Geometry: final body of the model. Coordinates: model frame, mm. Give positions to 0.01 mm unless a question says otherwise; leave off trailing zeros. Loops run counter-clockwise (first coordinate to the right, second up) from the corner with the lowest first, then second, coordinate; pieces in that order, holes last. Notation, with made-up numbers: (34, 78) -> (68, 78) arc R11 cw to (68, 83) -> close; hole circle Ø2 at (33, 46.25). An arc over 180 degrees is marked (long way). Answer in a Markdown table with one row per item. Add a question column.
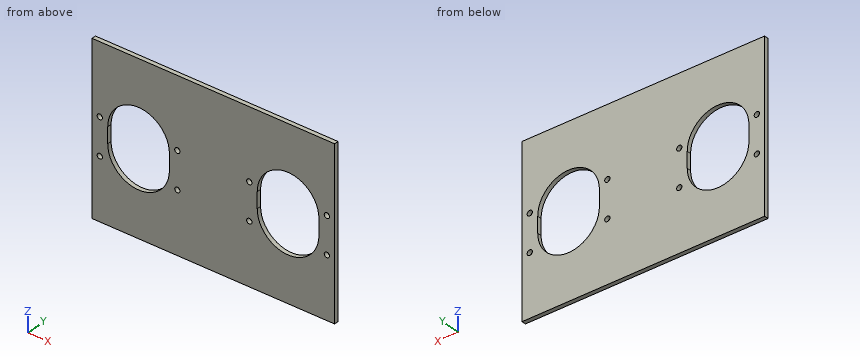
from build123d import *

# Parameters (mm, degrees)
F0_W     = 688
F0_H     = 90
F0_H_2   = 300
F0_R     = 7.5
F1_DEPTH = 12


with BuildPart() as f1:
    # F0 (on Front) → F1 (new body)
    with BuildSketch(Plane.XZ):
        with Locations((344, 345)):
            Rectangle(F0_W, F0_H)
        with Locations((344, 150)):
            Rectangle(F0_W, F0_H_2)
        with Locations((22, 85)):
            Circle(F0_R, mode=Mode.SUBTRACT)
        with Locations((242, 85)):
            Circle(F0_R, mode=Mode.SUBTRACT)
        with Locations((446, 85)):
            Circle(F0_R, mode=Mode.SUBTRACT)
        with Locations((666, 85)):
            Circle(F0_R, mode=Mode.SUBTRACT)
        with Locations((22, 190)):
            Circle(F0_R, mode=Mode.SUBTRACT)
        with BuildLine():
            ThreePointArc((44.5, 172.5), (132, 260), (219.5, 172.5))
            Line((219.5, 172.5), (219.5, 127.5))
            ThreePointArc((219.5, 127.5), (132, 40), (44.5, 127.5))
            Line((44.5, 127.5), (44.5, 172.5))
        make_face(mode=Mode.SUBTRACT)
        with Locations((242, 190)):
            Circle(F0_R, mode=Mode.SUBTRACT)
        with Locations((446, 190)):
            Circle(F0_R, mode=Mode.SUBTRACT)
        with BuildLine():
            ThreePointArc((468.5, 172.5), (556, 260), (643.5, 172.5))
            Line((643.5, 172.5), (643.5, 127.5))
            ThreePointArc((643.5, 127.5), (556, 40), (468.5, 127.5))
            Line((468.5, 127.5), (468.5, 172.5))
        make_face(mode=Mode.SUBTRACT)
        with Locations((666, 190)):
            Circle(F0_R, mode=Mode.SUBTRACT)
        with Locations((344, -45)):
            Rectangle(F0_W, F0_H)
    extrude(amount=F1_DEPTH)


solid = f1.part
(1) Cut plane C-C on y = -5.75. State how many separate pieces and enclosed holes the cut face has, then the cut area to 3 significant figures.
(2) Material intervals for line 1 along Z through (x, y) = (242, -5.75); line 2 along X through (y, z) = (-9.5, 128); line 3 along X through (y, z) = (-10, 124.5), sorted ascending. Write a range as from..to.
(3) Pin query (flat end, axial travel): pin 1 Ø9 at (x, z) = (242, 190) entering from +Y; pin 2 Ø19.5 at (x, z) = (22, 85) entering from +Y. Return the tip coordinate at first contact, or that it passes through.
(4) Cut plane A-A on x = 22. Return the cut outline in (y, z), then the cut area to 3 significant figures.
(5) Cut plane D-D on x = 200.5. Return the cut outline in (y, z).
(6) Cut plane B-B on z = 114. Return the cut outline in (x, y).
Answer list:
| question | item | result |
|---|---|---|
| 1 | separate pieces | 1 |
| 1 | enclosed holes | 10 |
| 1 | area | 265,000 mm² |
| 2 | line 1 | z = -90..77.5, 92.5..182.5, 197.5..390 |
| 2 | line 2 | x = 0..44.5, 219.5..468.5, 643.5..688 |
| 2 | line 3 | x = 0..44.55, 219.45..468.55, 643.45..688 |
| 3 | pin 1 | passes through |
| 3 | pin 2 | stops at y = 0 |
| 4 | outline | (-12, -90) -> (0, -90) -> (0, 77.5) -> (-12, 77.5) -> close; (-12, 92.5) -> (0, 92.5) -> (0, 182.5) -> (-12, 182.5) -> close; (-12, 197.5) -> (0, 197.5) -> (0, 390) -> (-12, 390) -> close |
| 4 | area | 5,400 mm² |
| 5 | outline | (-12, -90) -> (0, -90) -> (0, 73.06) -> (-12, 73.06) -> close; (-12, 226.94) -> (0, 226.94) -> (0, 390) -> (-12, 390) -> close |
| 6 | outline | (0, -12) -> (45.55, -12) -> (45.55, 0) -> (0, 0) -> close; (218.45, -12) -> (469.55, -12) -> (469.55, 0) -> (218.45, 0) -> close; (642.45, -12) -> (688, -12) -> (688, 0) -> (642.45, 0) -> close |
